from build123d import *

# Parameters (mm, degrees)
F0_W      = 508
F0_H      = 508
F4_T      = -2.54
F7_DEPTH  = 25.4
F10_DEPTH = 25.4
F13_DEPTH = 25.4
F16_DEPTH = 25.4


with BuildPart() as f3:
    # F0 (on Front) → F3 section 0
    with BuildSketch(Plane.XZ, mode=Mode.PRIVATE) as f3_s0:
        with Locations((-254, 254)):
            Rectangle(F0_W, F0_H)
    loft([f3_s0.sketch, Vertex(-254, -1270, 254)])

    # F4
    f4_openings = [f3.faces().sort_by_distance(p)[0] for p in [
        (-254, 0, 254),
    ]]
    offset(amount=F4_T, openings=f4_openings)

    # F6 (on offset) → F7 (cut)
    with BuildSketch(Plane(origin=(0, 0, 0), x_dir=(0.1961161351, 0.9805806757, 0), z_dir=(0.9805806757, -0.1961161351, 0))):
        Polygon((-25.4, 31.1354669124), (-25.4, 488.3354669124), (-1168.4, 259.7354669124), align=None)
    extrude(amount=-F7_DEPTH, mode=Mode.SUBTRACT)

    # F9 (on offset) → F10 (cut)
    with BuildSketch(Plane(origin=(-488.4615384615, -97.6923076923, 0), x_dir=(0.1961161351, -0.9805806757, 0), z_dir=(-0.9805806757, -0.1961161351, 0))):
        Polygon((813.1548545488, 310.3141247361), (-73.7252337318, 487.6901423922), (-73.7252337318, 254), (1043.8240543072, 254), (1059.226906247, 257.080570388), align=None)
        Polygon((1043.8240543072, 254), (-73.7252337318, 254), (-73.7252337318, 30.4901423922), align=None)
    extrude(amount=-F10_DEPTH, mode=Mode.SUBTRACT)

    # F12 (on offset) → F13 (cut)
    with BuildSketch(Plane(origin=(0, -97.6923076923, 488.4615384615), x_dir=(1, 0, 0), z_dir=(0, -0.1961161351, 0.9805806757))):
        Polygon((-247.3090775045, -1059.2242055456), (-19.3738871979, 80.4517459869), (-254, 80.4517459869), (-254, -1025.7695930679), align=None)
        Polygon((-254, 80.4517459869), (-475.244267811, 80.4517459869), (-254, -1025.7695930679), align=None)
    extrude(amount=-F13_DEPTH, mode=Mode.SUBTRACT)

    # F15 (on offset) → F16 (cut)
    with BuildSketch(Plane(origin=(0, 0, 0), x_dir=(1, 0, 0), z_dir=(0, -0.1961161351, -0.9805806757))):
        Polygon((-44.116795063, 31.3945114613), (-260.3600621223, 1206.6667079926), (-476.6033291817, 31.3945114613), align=None)
    extrude(amount=-F16_DEPTH, mode=Mode.SUBTRACT)


solid = f3.part
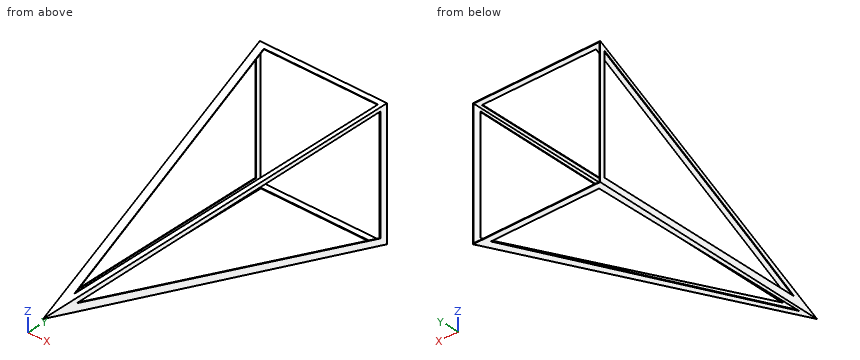
Work out the finished part from the listing and answer in its coordinate system (mm). Give positions to 0.01 mm unless a question says otherwise; leave off trailing zeros. Loops run counter-clockwise (first coordinate to the right, second up) from the corner with the lowest first, then second, coordinate; pieces in that order, holes last. Notation, with made-up numbers: (25.5, 45) -> (71.5, 45) arc R20 ccw to (71.5, 76) -> close; hole circle Ø8 at (18.25, 32.5). An arc over 180 degrees is marked (long way). Use a Markdown table: item, result. Add a question column.
1. Section C-C on x = -451.5 is taken. Determine the outline of the cut face in (y, z), and give its area (3 significant figures).
2. Flat-ended cylindrical pins translate along their axes: pin 1 Ø12 at (x, y) = (-150, -593.5) entering from -Z; pin 2 Ø3 at (y, z) = (-706, 367.5) entering from +X; pin 3 Ø2 at (x, y) = (-158.5, -792) entering from +Z. Find the tip coordinate at first contact, or state that the pin passes through.
3. Section A-A on z = 192 is taken. Determine the outline of the cut face in (x, y).
4. Find the intervals of material crossed by probe 1 along Z at (x, y) = (-464.5, -194), in increasing order.
5. Section B-B on y = -77 is taken. Determine the outline of the cut face in (x, z), and give its area (3 significant figures).
6. Section D-D on y = -971 is taken. Determine the outline of the cut face in (x, z), and give its area (3 significant figures).
Results below:
| question | item | result |
|---|---|---|
| 1 | outline | (-282.5, 56.5) -> (-164.57, 32.91) -> (-164.07, 35.4) -> (-269.55, 56.5) -> (-269.55, 80.39) -> (-282.5, 82.93) -> close; (-282.5, 435.25) -> (-269.55, 437.79) -> (-269.55, 451.5) -> (-134.72, 478.47) -> (-135.22, 480.96) -> (-282.5, 451.5) -> close; (-30.78, 6.16) -> (0, 0) -> (0, 2.59) -> (-30.29, 8.65) -> close; (-18.8, 504.24) -> (-18.3, 501.75) -> (0, 505.41) -> (0, 508) -> close |
| 1 | area | 1,300 mm^2 |
| 2 | pin 1 | stops at z = 117.53 |
| 2 | pin 2 | stops at x = -140.91 |
| 2 | pin 3 | stops at z = 349.8 |
| 3 | outline | (-508, 0) -> (-502.92, -25.4) -> (-500.43, -24.9) -> (-505.41, 0) -> close; (-344.55, -817.27) -> (-316, -960) -> (-302.25, -960) -> (-304.58, -947.05) -> (-316, -947.05) -> (-342.06, -816.77) -> close; (-218.47, -960) -> (-192, -960) -> (-162.72, -813.61) -> (-165.21, -813.11) -> (-192, -947.05) -> (-216.14, -947.05) -> close; (-7.47, -24.41) -> (-4.98, -24.91) -> (0, 0) -> (-2.59, 0) -> close |
| 4 | probe 1 | z = 38.8 to 41.39, 466.61 to 469.2 |
| 5 | outline | (-492.6, 15.4) -> (-467.93, 15.4) -> (-467.84, 17.99) -> (-490.01, 17.99) -> (-490.01, 41.12) -> (-492.6, 41.01) -> close; (-492.6, 477.17) -> (-490.01, 477.06) -> (-490.01, 490.01) -> (-463.27, 490.01) -> (-463.37, 492.6) -> (-492.6, 492.6) -> close; (-52.88, 17.99) -> (-52.79, 15.4) -> (-15.4, 15.4) -> (-15.4, 41.76) -> (-17.99, 41.86) -> (-17.99, 17.99) -> close; (-31.35, 490.01) -> (-17.99, 490.01) -> (-17.99, 477.61) -> (-15.4, 477.71) -> (-15.4, 492.6) -> (-31.24, 492.6) -> close |
| 5 | area | 465 mm^2 |
| 6 | outline | (-313.8, 194.2) -> (-300.18, 194.2) -> (-300.09, 196.79) -> (-311.21, 196.79) -> (-311.21, 223.46) -> (-313.8, 223.36) -> close; (-313.8, 293.56) -> (-311.21, 293.45) -> (-311.21, 311.21) -> (-280.93, 311.21) -> (-281.03, 313.8) -> (-313.8, 313.8) -> close; (-220.63, 196.79) -> (-220.54, 194.2) -> (-194.2, 194.2) -> (-194.2, 224.1) -> (-196.79, 224.2) -> (-196.79, 196.79) -> close; (-213.69, 311.21) -> (-196.79, 311.21) -> (-196.79, 295.27) -> (-194.2, 295.37) -> (-194.2, 313.8) -> (-213.58, 313.8) -> close |
| 6 | area | 466 mm^2 |
